from build123d import *

# Parameters (mm, degrees)
SKETCH_1_W          = 160
SKETCH_1_H          = 130
EXTRUDE_1_DEPTH     = 10
CUT_EXTRUDE_1_DEPTH = 10
EXTRUDE_2_DEPTH     = 25


with BuildPart() as part:
    # 草图1 → 凸台-拉伸1 (new body)
    with BuildSketch(Plane.XY):
        Rectangle(SKETCH_1_W, SKETCH_1_H)
    extrude(amount=EXTRUDE_1_DEPTH)

    # 草图2 → 切除-拉伸1 (cut)
    with BuildSketch(Plane.XY.offset(10)):
        Polygon((-32.5, 35), (-32.5, 65), (32.5, 65), (32.5, 35), (32.5, -35), (-32.5, -35), align=None)
    extrude(amount=-CUT_EXTRUDE_1_DEPTH, mode=Mode.SUBTRACT)

    # 草图3 → 凸台-拉伸2 (add)
    with BuildSketch(Plane.XY.offset(10)):
        Polygon((-70, 65), (-70, -55), (70, -55), (70, 65), (80, 65), (80, -65), (-80, -65), (-80, 65), align=None)
    extrude(amount=EXTRUDE_2_DEPTH)


solid = part.part
Part model, mm, in its own coordinate system. A direction names the side the tool comes from. Coordinates: 2 decimals unless noted, no trailing zeros. Loops run counter-clockwise (first coordinate to the right, second up) from the corner with the lowest first, then second, coordinate; pieces in that order, holes last. Notation, with made-up numbers: (62, 46) -> (117, 46) arc R38 ccw to (117, 85) -> close; hole circle Ø9 at (-14, 82.5). An arc over 180 degrees is marked (long way). Use a Markdown table: item, result. Add a question column.
Item 1: Probe probe 1 along X at (y, z) = (-8, 25); probe 2 along X at (y, z) = (2.5, 8); probe 3 along Z at (x, y) = (50, -38). List the from-to ranges inside material, lowest first.
Item 2: Flat gauge pin, fed straight in: P1, Ø8, axis at x = -12, z = 6, coming from the +Y side. Where does the tip first touch, or does it go through?
Item 3: Band-saw the part on C-C on y = -37. Write the cut outline in (x, z), plus the area to 3 significant figures.
Item 4: Band-saw the part on D-D on x = 13. Write the cut outline in (y, z).
Item 5: Band-saw the part on B-B on z = 6. Write the cut outline in (x, y), plus the area to 3 significant figures.
Item 6: Which spindle directions (+Z, -Z, +X, -X, +Y, -Y) get a long thin tool onto all of the face, cutting with end or side? Do faces 5 (the flat face through (-37, 1, 0)), 6 (the flat face through (70, 4, 22)), 7 (the flat face through (-32.5, 16, 5)). Say none if no direction does.
Item 7: Pull direction X, two halves, no side cores. Call faces 1 (the flat face through (0, -57, 35)), 2 (the flat face through (-1, -47, 10)), 3 (the flat face through (-80, -1, 17)), 4 (the flat face through (80, 1, 17)): +X half, -X half, draft (parallel to the pull), parting line (faces both ways), or undercut.
Item 8: Band-saw the part on A-A on y = 28. Write the cut outline in (x, z).
Geometry says:
| question | item | result |
|---|---|---|
| 1 | probe 1 | -80 to -70, 70 to 80 |
| 1 | probe 2 | -80 to -32.5, 32.5 to 80 |
| 1 | probe 3 | 0 to 10 |
| 2 | P1 | y = -35 |
| 3 | outline | (-80, 0) -> (80, 0) -> (80, 35) -> (70, 35) -> (70, 10) -> (-70, 10) -> (-70, 35) -> (-80, 35) -> close |
| 3 | area | 2,100 mm² |
| 4 | outline | (-65, 0) -> (-35, 0) -> (-35, 10) -> (-55, 10) -> (-55, 35) -> (-65, 35) -> close |
| 5 | outline | (-80, -65) -> (80, -65) -> (80, 65) -> (32.5, 65) -> (32.5, -35) -> (-32.5, -35) -> (-32.5, 65) -> (-80, 65) -> close |
| 5 | area | 14,300 mm² |
| 6 | face 5 | -Z, +X, -X, +Y, -Y |
| 6 | face 6 | +Z, +Y |
| 6 | face 7 | +Z, -Z, +Y |
| 7 | face 1 | draft |
| 7 | face 2 | undercut |
| 7 | face 3 | -X half |
| 7 | face 4 | +X half |
| 8 | outline | (-80, 0) -> (-32.5, 0) -> (-32.5, 10) -> (-70, 10) -> (-70, 35) -> (-80, 35) -> close; (32.5, 0) -> (80, 0) -> (80, 35) -> (70, 35) -> (70, 10) -> (32.5, 10) -> close |
